Input: dimensioned drawing with shaded views. Units: mm. Origin: part minimum x, y, z. A direction names the side the tool comes from. Round coordinates to 2 decimals unless told otherwise and drop trailing zeros. Loops run counter-clockwise (first coordinate to the right, second up) from the corner with the lowest first, then second, coordinate; pieces in that order, holes last. Notation, with made-up numbers: (-2.5, -34) - (21.5, -34) arc R10 ccw to (21.5, -20) - close; hole circle Ø1 at (46, 55). An arc over 180 degrees is marked (long way). One line per question, with ' | ' between items. Start each with the question number.
1. Mould query, pull axis X, two halves, no side actions, for the marked faces 4, 5 and 6. Classes: pulls with the +X half, pulls with the -X half, needs draft (parallel to the pull), parting line crosses it, or undercut.
2. Pin query (flat end, axial travel): pin 1 (5 mm diameter, centred on x = 17, z = 24, fed in from -Y); pin 2 (8.5 mm diameter, centred on x = 48, y = 74.5, fed in from +Z); pin 3 (10 mm diameter, centred on x = 37.5, z = 21.5, fed in from -Y); pin 4 (3 mm diameter, centred on x = 52.5, z = 19.5, fed in from +Y). Return the tip coordinate at first contact, or that it passes through.
3. Cut plane D-D (z = 22). Return loops of the section in (x, y).
4. Access query for the marked faces 1, 2 and 3. Directions: +Z, -Z, +X, -X, +Y, -Y. A direction counts if a zero-diameter tool reaches every point of the face in a straight line with its end or side. Return the directions, or none.
5. Cut plane C-C (z = 32). Return loops of the section in (x, y), then the cut area to 3 significant figures.
6. Ray query, line 1 (Y direction, x = 41, z = 37) (1 decimal); line 2 (X direction, y = 48.5, z = 14.5); line 3 (Y direction, x = 44.5, z = 23.5). Return the intervals inside material, ascending.
7. Cut plane A-A (x = 48). State how many separate pieces and enclosed holes the cut face has, then the cut area to 3 significant figures.
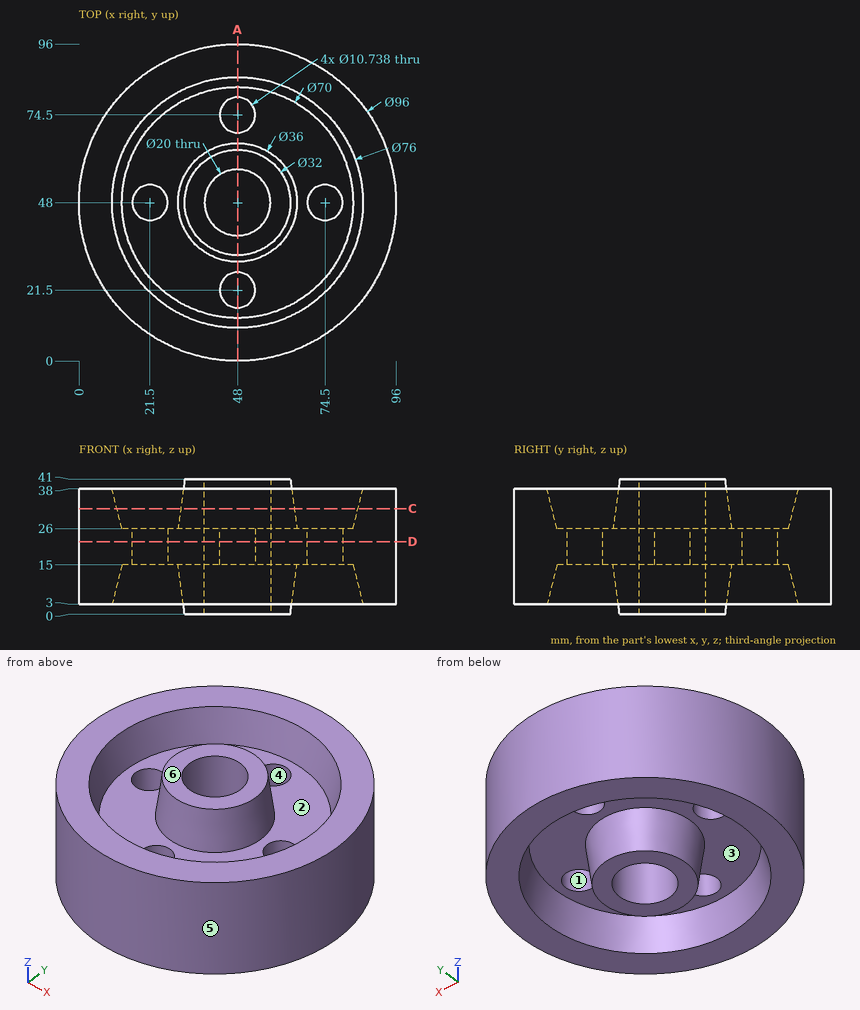
Answers follow:
1) face 4: undercut | face 5: parting line crosses it | face 6: needs draft
2) pin 1: stops at y = 9.38 | pin 2: passes through | pin 3: stops at y = 0.32 | pin 4: stops at y = 95.91
3) outline: circle Ø96 at (48, 48); hole circle Ø10.74 at (21.5, 48); hole circle Ø20 at (48, 48); hole circle Ø10.74 at (48, 21.5); hole circle Ø10.74 at (48, 74.5); hole circle Ø10.74 at (74.5, 48)
4) face 1: +Z, -Z | face 2: +Z | face 3: -Z
5) outline: circle Ø96 at (48, 48); circle Ø34.4 at (48, 48); hole circle Ø73 at (48, 48); hole circle Ø20 at (48, 48) | area: 3,670 mm2
6) line 1: y = 0.5 to 10.9, 33 to 40.9, 55.1 to 63, 85.1 to 95.5 | line 2: x = 0 to 12.88, 30.07 to 38.01, 57.99 to 65.93, 83.12 to 96 | line 3: y = 0.13 to 17.43, 25.57 to 38.63, 57.37 to 70.43, 78.57 to 95.87
7) separate pieces: 4 | enclosed holes: 0 | area: 1,570 mm2
